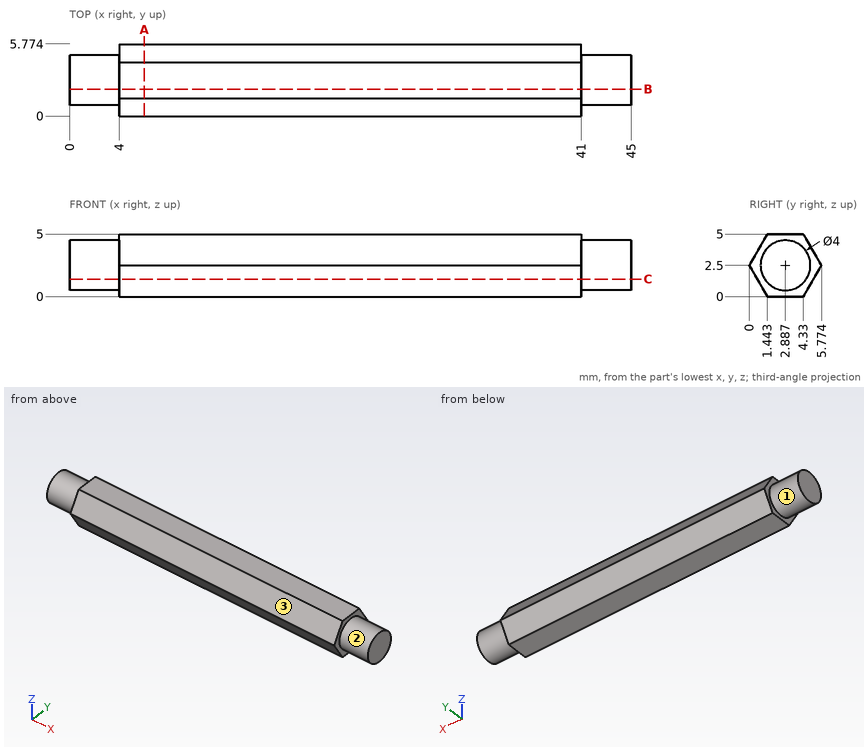
Part print with two shaded views. Sizes in mm from the minimum x, y, z corner. A direction names the side the tool comes from. Give positions to 0.01 mm unless a question says otherwise; leave off trailing zeros. Order: outer loops, then holes, each group sorted by start corner. A loop starts at its lowest first (then second) coordinate and runs counter-clockwise, first axis right, second up.
1) 3-axis set-ups, long thin cutter, end or side, ignore diameter. For the marked faces 1, 2 and 3: which of +Z, -Z, +X, -X, +Y, -Y reach the whole face in a straight line?
2) Saw through at A-A, the plane x = 6. Write the cut outline in (y, z).
3) Pin check, flat tip, straight feed: pin 1 (3 mm diameter, centred on x = 23, z = 0.5, fed in from +Y) (1 decimal). Stop position of the tip, or through.
4) Wall check: probe 1 along X at (y, z) = (4.4, 1.1); probe 2 along Y at (x, z) = (33.5, 3.4) (1 decimal); probe 3 along Z at (x, y) = (2, 2.25) (1 decimal). Give the ranges that are in metal, low to high.
5) Saw through at B-B, the plane y = 2.15. Write the cut outline in (x, z), then the cut area to 3 significant figures.
6) Saw through at C-C, the plane z = 1.4. Write the cut outline in (x, y) (1 decimal).
Computed:
1. face 1: -X
1. face 2: +X
1. face 3: +Z, +X, -X, -Y
2. outline: (0, 2.5) - (1.44, 0) - (4.33, 0) - (5.77, 2.5) - (4.33, 5) - (1.44, 5) - close
3. pin 1: stops at y = 5.5
4. probe 1: x = 4 to 41
4. probe 2: y = 0.5 to 5.3
4. probe 3: z = 0.6 to 4.4
5. outline: (0, 0.64) - (4, 0.64) - (4, 0) - (41, 0) - (41, 0.64) - (45, 0.64) - (45, 4.36) - (41, 4.36) - (41, 5) - (4, 5) - (4, 4.36) - (0, 4.36) - close
5. area: 215 mm2
6. outline: (0, 1.2) - (4, 1.2) - (4, 0.6) - (41, 0.6) - (41, 1.2) - (45, 1.2) - (45, 4.6) - (41, 4.6) - (41, 5.1) - (4, 5.1) - (4, 4.6) - (0, 4.6) - close
